Build history of the part. All positions in model axes, mm. Give positions to 0.01 mm unless a question says otherwise; leave off trailing zeros. Order: outer loops, then holes, each group sorted by start corner. A loop starts at its lowest first (then second) coordinate and runs counter-clockwise, first axis right, second up. Notation, with made-up numbers: M 11.25,85.25 L 69.25,85.25 A25 ccw 69.25,99.25 Z; hole C -32,17 d5. An arc over 180 degrees is marked long. Use CSV: the item, a comma, the result in double quotes. Start each with the question number.
Item 1: Band-saw the part on C-C on y = 1. Write the cut outline in (x, z).
Item 2: Band-saw the part on A-A on x = 0. Give the number of separate pieces and of enclosed holes in the cut face, plus the area to 3 significant figures.
Item 3: Band-saw the part on D-D on x = -18. Write the cut outline in (y, z).
Item 4: Pin check, flat tips, straight feed: P1, Ø10, axis at x = -15.875, y = 0, coming from the +Z side; P2, Ø8, axis at x = -13, z = 11.5, coming from the -Y side; P3, Ø10, axis at x = -7.5, z = 18.5, coming from the +Y side. Stop position of each tip, or through.
Item 5: Two-plate mould, pull along X, no slides. Class faces 1 (the cylindrical face through (-3.78, -2.9, 19.32)), 2 (the cylindrical face through (-7.559, -5.796, 31.661)), 3 (the flat face through (0, -10, 25.4)): pulls with the +X half, pulls with the -X half, needs draft (parallel to the pull), parting line crosses it, or undercut.
Item 6: Wall check: line 1 along Y through (x, z) = (1.5, 16.5); line 2 along Z through (x, y) = (2.5, -10); line 3 along X through (y, z) = (-1, 16). Give the ranges that are in metal, low to high.
from build123d import *

# Parameters (mm, degrees)
F0_R     = 22.225
F0_R_2   = 9.525
F1_DEPTH = 25.4
F0_R_3   = 4.7625
F2_DEPTH = 38.1
F3_R     = 4.7625
F4_DEPTH = 38.1


with BuildPart() as f1:
    # F0 (on Top) → F1 (new body)
    with BuildSketch(Plane.XY):
        Circle(F0_R)
        with BuildLine():
            ThreePointArc((3.159085, 15.5575), (11.22532, 11.22532), (15.5575, 3.159085))
            ThreePointArc((15.5575, 3.159085), (18.004855, 2.354643), (19.05, 0))
            ThreePointArc((19.05, 0), (18.004855, -2.354643), (15.5575, -3.159085))
            ThreePointArc((15.5575, -3.159085), (11.22532, -11.22532), (3.159085, -15.5575))
            ThreePointArc((3.159085, -15.5575), (3.171019, -15.716051), (3.175, -15.875))
            ThreePointArc((3.175, -15.875), (-0.158949, -19.046019), (-3.159085, -15.5575))
            ThreePointArc((-3.159085, -15.5575), (-11.22532, -11.22532), (-15.5575, -3.159085))
            ThreePointArc((-15.5575, -3.159085), (-19.05, 0), (-15.5575, 3.159085))
            ThreePointArc((-15.5575, 3.159085), (-11.22532, 11.22532), (-3.159085, 15.5575))
            ThreePointArc((-3.159085, 15.5575), (-0.158949, 19.046019), (3.175, 15.875))
            ThreePointArc((3.175, 15.875), (3.171019, 15.716051), (3.159085, 15.5575))
        make_face(mode=Mode.SUBTRACT)
        with BuildLine():
            ThreePointArc((15.5575, -3.159085), (12.7, 0), (15.5575, 3.159085))
            ThreePointArc((15.5575, 3.159085), (11.22532, 11.22532), (3.159085, 15.5575))
            ThreePointArc((3.159085, 15.5575), (0, 12.7), (-3.159085, 15.5575))
            ThreePointArc((-3.159085, 15.5575), (-11.22532, 11.22532), (-15.5575, 3.159085))
            ThreePointArc((-15.5575, 3.159085), (-13.520357, 2.129855), (-12.7, 0))
            ThreePointArc((-12.7, 0), (-13.520357, -2.129855), (-15.5575, -3.159085))
            ThreePointArc((-15.5575, -3.159085), (-11.22532, -11.22532), (-3.159085, -15.5575))
            ThreePointArc((-3.159085, -15.5575), (0, -12.7), (3.159085, -15.5575))
            ThreePointArc((3.159085, -15.5575), (11.22532, -11.22532), (15.5575, -3.159085))
        make_face()
        Circle(F0_R_2, mode=Mode.SUBTRACT)
    extrude(amount=F1_DEPTH)

    # F0 (on Top) → F2 (join)
    with BuildSketch(Plane.XY):
        Circle(F0_R_2)
        Circle(F0_R_3, mode=Mode.SUBTRACT)
        Circle(F0_R_3)
    extrude(amount=F2_DEPTH)

    # F3 (on face) → F4 (cut)
    with BuildSketch(Plane.XY.offset(38.1)):
        Circle(F3_R)
    extrude(amount=-F4_DEPTH, mode=Mode.SUBTRACT)


solid = f1.part
Model answer:
1,outline,"M -22.2,0 L -18.89,0 L -18.89,25.4 L -22.2,25.4 Z; M -12.86,0 L -4.66,0 L -4.66,38.1 L -9.47,38.1 L -9.47,25.4 L -12.86,25.4 Z; M 4.66,0 L 12.86,0 L 12.86,25.4 L 9.47,25.4 L 9.47,38.1 L 4.66,38.1 Z; M 18.89,0 L 22.2,0 L 22.2,25.4 L 18.89,25.4 Z"
2,separate pieces,"4"
2,enclosed holes,"0"
2,area,"685 mm^2"
3,outline,"M -13.04,0 L -2.36,0 L -2.36,25.4 L -13.04,25.4 Z; M 2.36,0 L 13.04,0 L 13.04,25.4 L 2.36,25.4 Z"
4,P1,"stops at z = 25.4"
4,P2,"stops at y = -20.32"
4,P3,"stops at y = 22.08"
5,face 1,"undercut"
5,face 2,"parting line crosses it"
5,face 3,"needs draft"
6,line 1,"y = -22.17 to -18.67, -13.08 to -4.52, 4.52 to 13.08, 18.67 to 22.17"
6,line 2,"z = 0 to 25.4"
6,line 3,"x = -22.2 to -18.89, -12.86 to -4.66, 4.66 to 12.86, 18.89 to 22.2"
